The drawing under review shows one solid part. Ordinate dimensions are in mm from its lowest x, y, z. A direction names the side the tool comes from. Coordinates: 2 decimals unless noted, no trailing zeros. Write each loop counter-clockwise with the first axis right and the second up, starting at its lowest first coordinate (ties: lowest second). Pieces come first, ordered by that corner, then holes.
1) For P1, Ø1.5, axis at x = 14, z = 7.5, coming from the -Y side; P2, Ø1, axis at y = 5.5, z = 12, coming from the -X side; P3, Ø3, axis at x = 15, z = 2, coming from the +Y side, all flat-tipped, find the tip position at first contact; note any pin that passes through.
2) Mouldability with a two-part tool opening along Y and no side actions: class the marked faces 5, 6 and 7 as released by +Y, released by -Y, zero draft, split by the parting line, or undercut.
3) Add section A-A, the plane x = 10. State the section outline as (y, z) points.
4) For line 1 (Z direction, x = 4.5, y = 18.25); line 2 (Y direction, x = 12, z = 5.75); line 3 (Z direction, x = 5.25, y = 6.5), list the stretches that pass through material, from the lowest coordinate up.
5) Machinability: for the marked faces 1, 2, 3 and 4, which of the approach directions +Z, -Z, +X, -X, +Y, -Y give a long, thin tool a straight path to every point of the face, cutting with its end or side? Answer none if there is none.
6) Add section D-D, the plane x = 16.75. State the section outline as (y, z) points.
7) Add section B-B, the plane z = 12.5. State the section outline as (x, y) points, then the cut area to 3 significant figures.
8) Add section C-C, the plane y = 18. State the section outline as (x, z) points, then the cut area to 3 significant figures.
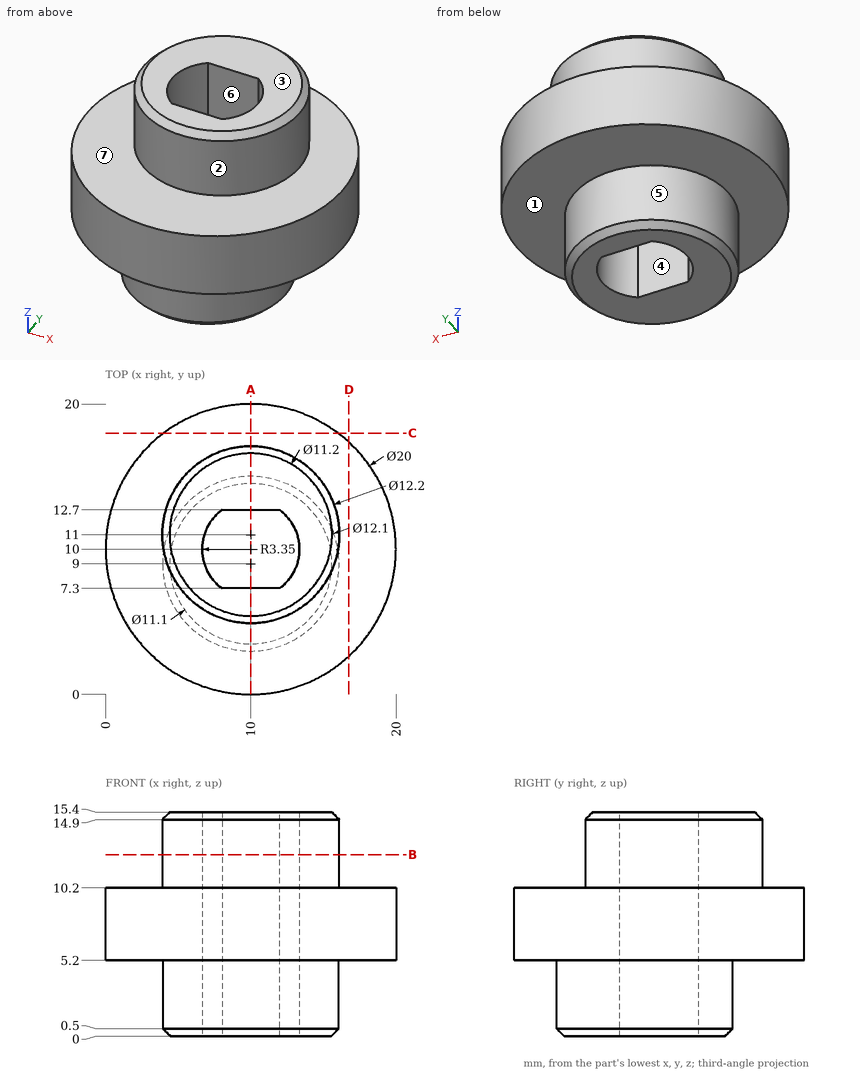
Geometry results:
1. P1: stops at y = 0.54
1. P2: stops at x = 6.51
1. P3: stops at y = 13.93
2. face 5: split by the parting line
2. face 6: undercut
2. face 7: zero draft
3. outline: (0, 5.2) - (2.95, 5.2) - (2.95, 0.5) - (3.45, 0) - (7.3, 0) - (7.3, 15.4) - (5.4, 15.4) - (4.9, 14.9) - (4.9, 10.2) - (0, 10.2) - close; (12.7, 0) - (14.55, 0) - (15.05, 0.5) - (15.05, 5.2) - (20, 5.2) - (20, 10.2) - (17.1, 10.2) - (17.1, 14.9) - (16.6, 15.4) - (12.7, 15.4) - close
4. line 1: z = 5.2 to 10.2
4. line 2: y = 0.2 to 7.31, 12.69 to 19.8
4. line 3: z = 0 to 10.2
5. face 1: -Z
5. face 2: +Z
5. face 3: +Z, +X, -X, +Y, -Y
5. face 4: +Z, -Z
6. outline: (2.62, 5.2) - (17.38, 5.2) - (17.38, 10.2) - (2.62, 10.2) - close
7. outline: circle Ø12.2 at (10, 11); hole (8.02, 7.3) - (11.98, 7.3) arc R3.35 ccw to (11.98, 12.7) - (8.02, 12.7) arc R3.35 ccw to start
7. area: 85.2 mm2
8. outline: (4, 5.2) - (16, 5.2) - (16, 10.2) - (4, 10.2) - close
8. area: 60.0 mm2
